Geometry check sheet. Reference: drawing and pictorial views, mm from the part's lowest x, y, z. Give positions to 0.01 mm unless a question says otherwise; leave off trailing zeros. Order: outer loops, then holes, each group sorted by start corner. A loop starts at its lowest first (then second) coordinate and runs counter-clockwise, first axis right, second up. Notation, with made-up numbers: M -37.5,-32 L 2.5,-32 A28 cw 2.5,-9 Z; hole C 16,-31.75 d10. An arc over 180 degrees is marked long. Answer as CSV lines item,"result".
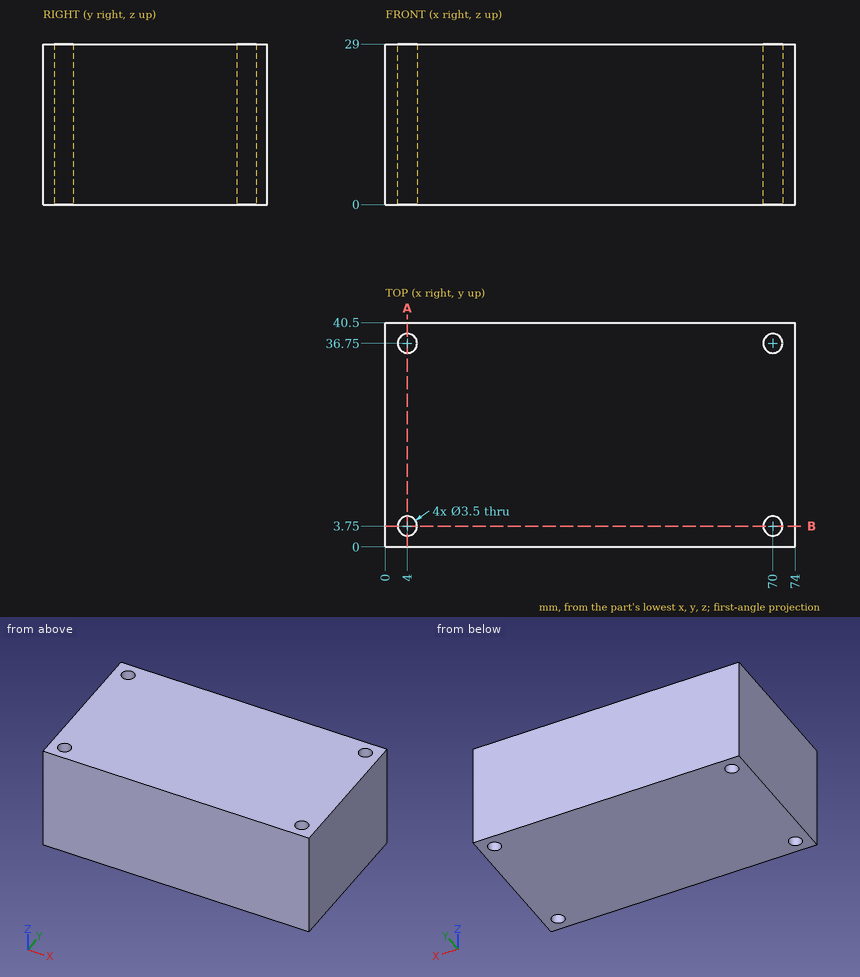
(1) Section check A-A on x = 4. Enter the section's corners in (y, z).
The answers:
outline,"M 0,0 L 2,0 L 2,29 L 0,29 Z; M 5.5,0 L 35,0 L 35,29 L 5.5,29 Z; M 38.5,0 L 40.5,0 L 40.5,29 L 38.5,29 Z"
(2) Material ranges on line 1 (X direction, y = 3.75, z = 22.5); line 2 (Y direction, x = 4, z = 15); line 3 (Y direction, x = 69.5, z = 12.75), recorded low to high.
The answers:
line 1,"x = 0 to 2.25, 5.75 to 68.25, 71.75 to 74"
line 2,"y = 0 to 2, 5.5 to 35, 38.5 to 40.5"
line 3,"y = 0 to 2.07, 5.43 to 35.07, 38.43 to 40.5"
(3) Section check B-B on y = 3.75. Enter the section's corners in (x, z).
The answers:
outline,"M 0,0 L 2.25,0 L 2.25,29 L 0,29 Z; M 5.75,0 L 68.25,0 L 68.25,29 L 5.75,29 Z; M 71.75,0 L 74,0 L 74,29 L 71.75,29 Z"
